The listing builds one solid part. Answer for the finished solid, in the listing's coordinates (mm). Face numbers are marked on the shaded views. A direction names the side the tool comes from. Coordinates: 2 decimals unless noted, no trailing zeros. Order: outer loops, then holes, each group sorted by start corner. A loop starts at its lowest first (then second) coordinate and runs counter-clockwise, first axis right, second up. Notation, with made-up numbers: (31.25, -2) - (45.25, -2) arc R7 cw to (45.25, 3) - close; hole circle Ø6 at (89.5, 19.5). An arc over 180 degrees is marked (long way). Use a Markdown table: item, result. Add a question column.
Item 1: The part is cut by section C-C, the plane y = 4. Give the vertices of the cut face in (x, z).
Item 2: The part is cut by section A-A, the plane x = 13.75. Give the vertices of the cut face in (y, z).
Item 3: The part is cut by section B-B, the plane z = 1.4. Give the vertices of the cut face in (x, y), then the cut area to 3 significant figures.
Item 4: Find the intervals of material crossed by line 1 along Y through (x, z) = (24, 2.4); line 2 along Y through (x, z) = (4, 0.9); line 3 along X through (y, z) = (4, 2.5), in increasing order.
Item 5: For the marked faces 4 and 5, determine the directions among +Z, -Z, +X, -X, +Y, -Y from which every point of the face is accessible in a straight line to the end or side of a thin tool.
Item 6: A flat-ended cylindrical pin translates along its axis: P1, Ø4, axis at x = 24, y = 4, coming from the -Z side. Find the tip coordinate at first contact, or state that the pin passes through.
Item 7: The mould has two halves that part along Y. Classify the marked faces 1, 2 and 3: released by +Y, released by -Y, zero draft, split by the parting line, or undercut.
Item 8: The part is cut by section D-D, the plane x = 4. Give the vertices of the cut face in (y, z).
from build123d import *

# Parameters (mm, degrees)
SKETCH1_W           = 28
SKETCH1_H           = 16
SKETCH1_R           = 1.2
SKETCH1_W_2         = 14
SKETCH1_H_2         = 2
BOSS_EXTRUDE1_DEPTH = 3.2
SKETCH2_R           = 3
CUT_EXTRUDE1_DEPTH  = 2.2


with BuildPart() as part:
    # Sketch1 → Boss-Extrude1 (new body)
    with BuildSketch(Plane.XY):
        with Locations((14, 8)):
            Rectangle(SKETCH1_W, SKETCH1_H)
        with Locations((4, 12)):
            Circle(SKETCH1_R, mode=Mode.SUBTRACT)
        with Locations(Location((4, 4, 0), (0, 0, 180))):
            Circle(SKETCH1_R, mode=Mode.SUBTRACT)
        with Locations((24, 4)):
            Circle(SKETCH1_R, mode=Mode.SUBTRACT)
        with Locations(Location((24, 12, 0), (0, 0, 180))):
            Circle(SKETCH1_R, mode=Mode.SUBTRACT)
        with Locations((14, 8)):
            Rectangle(SKETCH1_W_2, SKETCH1_H_2, mode=Mode.SUBTRACT)
    extrude(amount=BOSS_EXTRUDE1_DEPTH)

    # Sketch2 → Cut-Extrude1 (cut)
    with BuildSketch(Plane(origin=(0, 0, 0), x_dir=(-1, 0, 0), z_dir=(0, 0, -1))):
        with Locations((-4, 12)):
            Circle(SKETCH2_R)
        with Locations((-4, 4)):
            Circle(SKETCH2_R)
        with Locations((-24, 4)):
            Circle(SKETCH2_R)
        with Locations((-24, 12)):
            Circle(SKETCH2_R)
    extrude(amount=-CUT_EXTRUDE1_DEPTH, mode=Mode.SUBTRACT)


solid = part.part
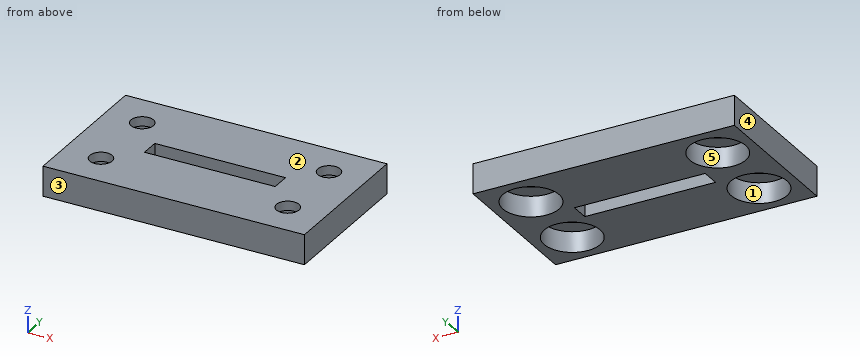
Solution:
| question | item | result |
|---|---|---|
| 1 | outline | (0, 0) - (1, 0) - (1, 2.2) - (2.8, 2.2) - (2.8, 3.2) - (0, 3.2) - close; (5.2, 2.2) - (7, 2.2) - (7, 0) - (21, 0) - (21, 2.2) - (22.8, 2.2) - (22.8, 3.2) - (5.2, 3.2) - close; (25.2, 2.2) - (27, 2.2) - (27, 0) - (28, 0) - (28, 3.2) - (25.2, 3.2) - close |
| 2 | outline | (0, 0) - (7, 0) - (7, 3.2) - (0, 3.2) - close; (9, 0) - (16, 0) - (16, 3.2) - (9, 3.2) - close |
| 3 | outline | (0, 0) - (28, 0) - (28, 16) - (0, 16) - close; hole circle Ø6 at (4, 4); hole circle Ø6 at (4, 12); hole (7, 7) - (21, 7) - (21, 9) - (7, 9) - close; hole circle Ø6 at (24, 4); hole circle Ø6 at (24, 12) |
| 3 | area | 307 mm2 |
| 4 | line 1 | y = 0 to 2.8, 5.2 to 10.8, 13.2 to 16 |
| 4 | line 2 | y = 0 to 1, 7 to 9, 15 to 16 |
| 4 | line 3 | x = 0 to 2.8, 5.2 to 22.8, 25.2 to 28 |
| 5 | face 4 | +Z, -Z, -X, +Y, -Y |
| 5 | face 5 | -Z |
| 6 | P1 | stops at z = 2.2 |
| 7 | face 1 | undercut |
| 7 | face 2 | zero draft |
| 7 | face 3 | released by -Y |
| 8 | outline | (0, 0) - (1, 0) - (1, 2.2) - (2.8, 2.2) - (2.8, 3.2) - (0, 3.2) - close; (5.2, 2.2) - (7, 2.2) - (7, 0) - (9, 0) - (9, 2.2) - (10.8, 2.2) - (10.8, 3.2) - (5.2, 3.2) - close; (13.2, 2.2) - (15, 2.2) - (15, 0) - (16, 0) - (16, 3.2) - (13.2, 3.2) - close |
